```python
from build123d import *

# Parameters (mm, degrees)
BOSS_EXTRU_1_DEPTH      = 15
CONG_1_R                = 2
ENL_V_MAT_EXTRU_1_REACH = 4
ESQUISSE2_R             = 2.5
ENL_V_MAT_EXTRU_2_REACH = 4
ESQUISSE4_R             = 2.5


with BuildPart() as part:
    # Esquisse1 → Boss.-Extru.1 (new body, symmetric)
    with BuildSketch(Plane(origin=(0, 0, 0), x_dir=(0, 0, -1), z_dir=(1, 0, 0))):
        Polygon((0, 0), (0, 100), (2, 100), (2, 2), (55, 2), (55, 0), align=None)
    extrude(amount=BOSS_EXTRU_1_DEPTH, both=True)

    # Congé1
    cong_1_edges = [part.edges().sort_by_distance(p)[0] for p in [
        (0, 0, 0),
        (0, 2, -2),
    ]]
    fillet(cong_1_edges, radius=CONG_1_R)

    # Esquisse2 → Enlèv. mat.-Extru.1 (cut, up to next)
    with BuildSketch(Plane(origin=(0, 2, 0), x_dir=(1, 0, 0), z_dir=(0, 1, 0)), mode=Mode.PRIVATE) as enl_v_mat_extru_1_sk1:
        with BuildLine():
            Line((4.25, 24.25), (4.25, 45.75))
            ThreePointArc((4.25, 45.75), (0, 50), (-4.25, 45.75))
            Line((-4.25, 45.75), (-4.25, 24.25))
            ThreePointArc((-4.25, 24.25), (0, 20), (4.25, 24.25))
        make_face()
    enl_v_mat_extru_1_tool1 = extrude(enl_v_mat_extru_1_sk1.sketch, amount=-ENL_V_MAT_EXTRU_1_REACH, mode=Mode.PRIVATE) & part.part
    add(enl_v_mat_extru_1_tool1.solids().sort_by_distance((0, 2, -35))[0], mode=Mode.SUBTRACT)
    # Esquisse2 → Enlèv. mat.-Extru.1 (cut, up to next)
    with BuildSketch(Plane(origin=(0, 2, 0), x_dir=(1, 0, 0), z_dir=(0, 1, 0)), mode=Mode.PRIVATE) as enl_v_mat_extru_1_sk2:
        with Locations((-9.5, 25)):
            Circle(ESQUISSE2_R)
    enl_v_mat_extru_1_tool2 = extrude(enl_v_mat_extru_1_sk2.sketch, amount=-ENL_V_MAT_EXTRU_1_REACH, mode=Mode.PRIVATE) & part.part
    add(enl_v_mat_extru_1_tool2.solids().sort_by_distance((-9.5, 2, -25))[0], mode=Mode.SUBTRACT)
    # Esquisse2 → Enlèv. mat.-Extru.1 (cut, up to next)
    with BuildSketch(Plane(origin=(0, 2, 0), x_dir=(1, 0, 0), z_dir=(0, 1, 0)), mode=Mode.PRIVATE) as enl_v_mat_extru_1_sk3:
        with Locations((-9.5, 45)):
            Circle(ESQUISSE2_R)
    enl_v_mat_extru_1_tool3 = extrude(enl_v_mat_extru_1_sk3.sketch, amount=-ENL_V_MAT_EXTRU_1_REACH, mode=Mode.PRIVATE) & part.part
    add(enl_v_mat_extru_1_tool3.solids().sort_by_distance((-9.5, 2, -45))[0], mode=Mode.SUBTRACT)
    # Esquisse2 → Enlèv. mat.-Extru.1 (cut, up to next)
    with BuildSketch(Plane(origin=(0, 2, 0), x_dir=(1, 0, 0), z_dir=(0, 1, 0)), mode=Mode.PRIVATE) as enl_v_mat_extru_1_sk4:
        with Locations((9.5, 45)):
            Circle(ESQUISSE2_R)
    enl_v_mat_extru_1_tool4 = extrude(enl_v_mat_extru_1_sk4.sketch, amount=-ENL_V_MAT_EXTRU_1_REACH, mode=Mode.PRIVATE) & part.part
    add(enl_v_mat_extru_1_tool4.solids().sort_by_distance((9.5, 2, -45))[0], mode=Mode.SUBTRACT)
    # Esquisse2 → Enlèv. mat.-Extru.1 (cut, up to next)
    with BuildSketch(Plane(origin=(0, 2, 0), x_dir=(1, 0, 0), z_dir=(0, 1, 0)), mode=Mode.PRIVATE) as enl_v_mat_extru_1_sk5:
        with Locations((9.5, 25)):
            Circle(ESQUISSE2_R)
    enl_v_mat_extru_1_tool5 = extrude(enl_v_mat_extru_1_sk5.sketch, amount=-ENL_V_MAT_EXTRU_1_REACH, mode=Mode.PRIVATE) & part.part
    add(enl_v_mat_extru_1_tool5.solids().sort_by_distance((9.5, 2, -25))[0], mode=Mode.SUBTRACT)

    # Esquisse4 → Enlèv. mat.-Extru.2 (cut, up to next)
    with BuildSketch(Plane(origin=(0, 0, -2), x_dir=(-1, 0, 0), z_dir=(0, 0, -1)), mode=Mode.PRIVATE) as enl_v_mat_extru_2_sk1:
        with Locations((-10, 85)):
            Circle(ESQUISSE4_R)
    enl_v_mat_extru_2_tool1 = extrude(enl_v_mat_extru_2_sk1.sketch, amount=-ENL_V_MAT_EXTRU_2_REACH, mode=Mode.PRIVATE) & part.part
    add(enl_v_mat_extru_2_tool1.solids().sort_by_distance((10, 85, -2))[0], mode=Mode.SUBTRACT)
    # Esquisse4 → Enlèv. mat.-Extru.2 (cut, up to next)
    with BuildSketch(Plane(origin=(0, 0, -2), x_dir=(-1, 0, 0), z_dir=(0, 0, -1)), mode=Mode.PRIVATE) as enl_v_mat_extru_2_sk2:
        with Locations((-10, 65)):
            Circle(ESQUISSE4_R)
    enl_v_mat_extru_2_tool2 = extrude(enl_v_mat_extru_2_sk2.sketch, amount=-ENL_V_MAT_EXTRU_2_REACH, mode=Mode.PRIVATE) & part.part
    add(enl_v_mat_extru_2_tool2.solids().sort_by_distance((10, 65, -2))[0], mode=Mode.SUBTRACT)
    # Esquisse4 → Enlèv. mat.-Extru.2 (cut, up to next)
    with BuildSketch(Plane(origin=(0, 0, -2), x_dir=(-1, 0, 0), z_dir=(0, 0, -1)), mode=Mode.PRIVATE) as enl_v_mat_extru_2_sk3:
        with Locations((-10, 45)):
            Circle(ESQUISSE4_R)
    enl_v_mat_extru_2_tool3 = extrude(enl_v_mat_extru_2_sk3.sketch, amount=-ENL_V_MAT_EXTRU_2_REACH, mode=Mode.PRIVATE) & part.part
    add(enl_v_mat_extru_2_tool3.solids().sort_by_distance((10, 45, -2))[0], mode=Mode.SUBTRACT)
    # Esquisse4 → Enlèv. mat.-Extru.2 (cut, up to next)
    with BuildSketch(Plane(origin=(0, 0, -2), x_dir=(-1, 0, 0), z_dir=(0, 0, -1)), mode=Mode.PRIVATE) as enl_v_mat_extru_2_sk4:
        with Locations((10, 75)):
            Circle(ESQUISSE4_R)
    enl_v_mat_extru_2_tool4 = extrude(enl_v_mat_extru_2_sk4.sketch, amount=-ENL_V_MAT_EXTRU_2_REACH, mode=Mode.PRIVATE) & part.part
    add(enl_v_mat_extru_2_tool4.solids().sort_by_distance((-10, 75, -2))[0], mode=Mode.SUBTRACT)
    # Esquisse4 → Enlèv. mat.-Extru.2 (cut, up to next)
    with BuildSketch(Plane(origin=(0, 0, -2), x_dir=(-1, 0, 0), z_dir=(0, 0, -1)), mode=Mode.PRIVATE) as enl_v_mat_extru_2_sk5:
        with Locations((10, 55)):
            Circle(ESQUISSE4_R)
    enl_v_mat_extru_2_tool5 = extrude(enl_v_mat_extru_2_sk5.sketch, amount=-ENL_V_MAT_EXTRU_2_REACH, mode=Mode.PRIVATE) & part.part
    add(enl_v_mat_extru_2_tool5.solids().sort_by_distance((-10, 55, -2))[0], mode=Mode.SUBTRACT)
    # Esquisse4 → Enlèv. mat.-Extru.2 (cut, up to next)
    with BuildSketch(Plane(origin=(0, 0, -2), x_dir=(-1, 0, 0), z_dir=(0, 0, -1)), mode=Mode.PRIVATE) as enl_v_mat_extru_2_sk6:
        with Locations((10, 35)):
            Circle(ESQUISSE4_R)
    enl_v_mat_extru_2_tool6 = extrude(enl_v_mat_extru_2_sk6.sketch, amount=-ENL_V_MAT_EXTRU_2_REACH, mode=Mode.PRIVATE) & part.part
    add(enl_v_mat_extru_2_tool6.solids().sort_by_distance((-10, 35, -2))[0], mode=Mode.SUBTRACT)
    # Esquisse4 → Enlèv. mat.-Extru.2 (cut, up to next)
    with BuildSketch(Plane(origin=(0, 0, -2), x_dir=(-1, 0, 0), z_dir=(0, 0, -1)), mode=Mode.PRIVATE) as enl_v_mat_extru_2_sk7:
        with BuildLine():
            Line((3.25, 90), (3.25, 30))
            ThreePointArc((3.25, 30), (0, 26.75), (-3.25, 30))
            Line((-3.25, 30), (-3.25, 90))
            ThreePointArc((-3.25, 90), (0, 93.25), (3.25, 90))
        make_face()
    enl_v_mat_extru_2_tool7 = extrude(enl_v_mat_extru_2_sk7.sketch, amount=-ENL_V_MAT_EXTRU_2_REACH, mode=Mode.PRIVATE) & part.part
    add(enl_v_mat_extru_2_tool7.solids().sort_by_distance((0, 60, -2))[0], mode=Mode.SUBTRACT)


solid = part.part
```
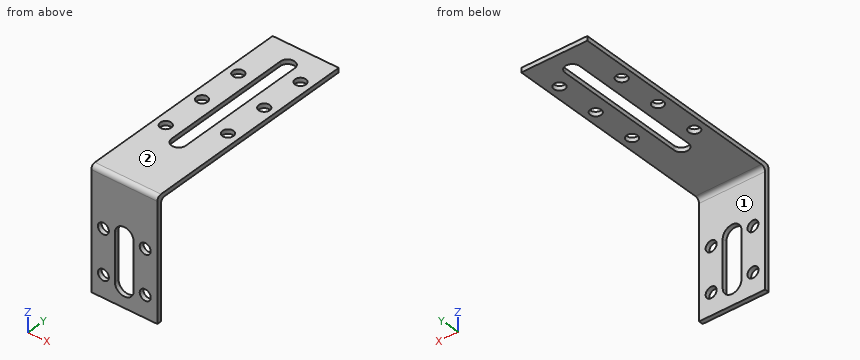
Build history of the part. All positions in model axes, mm. Face numbers are marked on the shaded views. A direction names the side the tool comes from. Give positions to 0.01 mm unless a question says otherwise; leave off trailing zeros. Order: outer loops, then holes, each group sorted by start corner. A loop starts at its lowest first (then second) coordinate and runs counter-clockwise, first axis right, second up. Notation, with made-up numbers: M 65.5,-3.75 L 111.5,-3.75 A23 cw 111.5,29.25 Z; hole C 47,65 d7. An arc over 180 degrees is marked long. Write item = value, one per line. Start each with the question number.
(1) Slice it at B-B on y = 55. Write the cut outline in (x, z), plus the area to 3 significant figures.
(2) Probe L1, parallel to Z at x = 9.5, y = 0.5; L2, parallel to Y at x = 10, z = -1.05; L3, parallel to Z at x = 9.5, y = 1.65. List the from-to ranges inside material, lowest first. Write a range as [from, to].
(3) Slice it at D-D on y = 81. Write the cut outline in (x, z), plus the area to 3 significant figures.
(4) Pin check, flat tips, straight feed: pin 1 Ø6.5 at (x, z) = (-9.5, -45) entering from +Y; pin 2 Ø12 at (x, y) = (5, 43) entering from -Z. Stop position of each tip, or through.
(5) Slice it at A-A on z = -34. Write the cut outline in (x, y).
(6) Slice it at C-C on x = 0. Write the cut outline in (y, z).
(7) Which spindle directions (+Z, -Z, +X, -X, +Y, -Y) get a long thin tool onto all of the face, cutting with end or side? Do the marked faces 1 and 2. Say none if no direction does.
Responses:
q1.outline = M -15,-2 L -12.5,-2 L -12.5,0 L -15,0 Z; M -7.5,-2 L -3.25,-2 L -3.25,0 L -7.5,0 Z; M 3.25,-2 L 15,-2 L 15,0 L 3.25,0 Z
q1.area = 37.0 mm2
q2.L1 = [-55, -47.5], [-42.5, -27.5], [-22.5, -0.68]
q2.L2 = [0.24, 42.5], [47.5, 62.5], [67.5, 82.5], [87.5, 100]
q2.L3 = [-55, -47.5], [-42.5, -27.5], [-22.5, -0.03]
q3.outline = M -15,-2 L -3.25,-2 L -3.25,0 L -15,0 Z; M 3.25,-2 L 15,-2 L 15,0 L 3.25,0 Z
q3.area = 47.0 mm2
q4.pin_1 = 2
q4.pin_2 = -2
q5.outline = M -15,0 L -4.25,0 L -4.25,2 L -15,2 Z; M 4.25,0 L 15,0 L 15,2 L 4.25,2 Z
q6.outline = M 0,-55 L 2,-55 L 2,-50 L 0,-50 Z; M 0,-20 L 2,-20 L 2,-4 A2 cw 4,-2 L 26.75,-2 L 26.75,0 L 2,0 A2 ccw 0,-2 Z; M 93.25,-2 L 100,-2 L 100,0 L 93.25,0 Z
q7.face_1 = -Z, +X, -X, +Y
q7.face_2 = +Z, +X, -X, +Y, -Y
